```python
from build123d import *

# Parameters (mm, degrees)
SKETCH2_W           = 80
SKETCH2_H           = 50
SKETCH2_R           = 3
BOSS_EXTRUDE1_DEPTH = 5
SKETCH3_R           = 2.5
CUT_EXTRUDE1_DEPTH  = 10


with BuildPart() as part:
    # Sketch2 → Boss-Extrude1 (new body)
    with BuildSketch(Plane(origin=(0, 0, 0), x_dir=(1, 0, 0), z_dir=(0, 1, 0))):
        with Locations((40, 25)):
            Rectangle(SKETCH2_W, SKETCH2_H)
        with Locations(Location((63.461538462, 10, 0), (0, 0, 270))):
            Circle(SKETCH2_R, mode=Mode.SUBTRACT)
        with Locations(Location((63.461538462, 40, 0), (0, 0, 270))):
            Circle(SKETCH2_R, mode=Mode.SUBTRACT)
    extrude(amount=BOSS_EXTRUDE1_DEPTH)

    # Sketch3 → Cut-Extrude1 (cut)
    with BuildSketch(Plane(origin=(0, 5, 0), x_dir=(1, 0, 0), z_dir=(0, 1, 0))):
        with Locations(Location((40.5, 7.5, 0), (0, 0, 270))):
            Circle(SKETCH3_R)
        with Locations(Location((9.5, 7.5, 0), (0, 0, 270))):
            Circle(SKETCH3_R)
        with Locations(Location((40.5, 42.5, 0), (0, 0, 270))):
            Circle(SKETCH3_R)
        with Locations(Location((9.5, 42.5, 0), (0, 0, 270))):
            Circle(SKETCH3_R)
    extrude(amount=-CUT_EXTRUDE1_DEPTH, mode=Mode.SUBTRACT)


solid = part.part
```
Check sheet for the modelled part. Datum: model origin and axes. Units: mm. Coordinates: 2 decimals unless noted, no trailing zeros. Write each loop counter-clockwise with the first axis right and the second up, starting at its lowest first coordinate (ties: lowest second). Pieces come first, ordered by that corner, then holes. Notation, with made-up numbers: M 27.5,-1 L 34.5,-1 A25 cw 34.5,37 Z; hole C -23.75,-26 d9. An arc over 180 degrees is marked long. Use one line per item in the form item = value.
Item 1: Gauge pin test, flat end, axial feed: pin 1 Ø5 at (x, z) = (63.46, -40) entering from -Y. Record the tip position at first contact, or that the pin passes through.
Answer below:
pin_1 = through
Item 2: Sectioned sample at A-A, the plane x = 9.5. Record the cut outline in (y, z), and give its area (3 significant figures).
Answer below:
outline = M 0,-50 L 5,-50 L 5,-45 L 0,-45 Z; M 0,-40 L 5,-40 L 5,-10 L 0,-10 Z; M 0,-5 L 5,-5 L 5,0 L 0,0 Z
area = 200 mm^2
Item 3: Release check for a two-part mould opening along X. For faces 1 (the face through (39, 2, 0)), 2 (the face through (0, 2, -25)), 3 (the face through (38.06, 2.54, -8.04)) record: pulls with the +X half, pulls with the -X half, needs draft (parallel to the pull), parting line crosses it, or undercut.
Answer below:
face_1 = needs draft
face_2 = pulls with the -X half
face_3 = undercut
Item 4: Sectioned sample at B-B, the plane y = 2.4. Record the cut outline in (x, z), and give its area (3 significant figures).
Answer below:
outline = M 0,-50 L 80,-50 L 80,0 L 0,0 Z; hole C 9.5,-42.5 d5; hole C 9.5,-7.5 d5; hole C 40.5,-42.5 d5; hole C 40.5,-7.5 d5; hole C 63.46,-40 d6; hole C 63.46,-10 d6
area = 3,860 mm^2
Item 5: Material ranges on L1, parallel to X at y = 3.85, z = -41.5; L2, parallel to X at y = 2.9, z = -7.5; L3, parallel to Z at x = 61, y = 4.7, recorded low to high. Write a range as from..to.
Answer below:
L1 = 0..7.21, 11.79..38.21, 42.79..60.86, 66.06..80
L2 = 0..7, 12..38, 43..61.8, 65.12..80
L3 = -50..-41.71, -38.29..-11.71, -8.29..0
